Part model, mm, in its own coordinate system. Face numbers are marked on the shaded views. A direction names the side the tool comes from. Give positions to 0.01 mm unless a question says otherwise; leave off trailing zeros. Order: outer loops, then holes, each group sorted by start corner. A loop starts at its lowest first (then second) coordinate and runs counter-clockwise, first axis right, second up.
1. Probe line 1 (Y direction, x = 8, z = 2); line 2 (Y direction, x = 31, z = 9); line 3 (X direction, y = -7.5, z = 8.75). List the from-to ranges inside material, lowest first.
2. Drop flat-ended pins along their axis: pin 1 Ø2.5 at (x, y) = (15, 0) entering from +Z; pin 2 Ø5 at (x, z) = (50, 2.5) entering from -Y; pin 3 Ø1 at (y, z) = (2.5, 7) entering from -X; pin 4 Ø1 at (y, z) = (4.5, 2) entering from -X. Give the stop position or say it passes through.
3. Slice it at B-B on y = 0. List the corners of the cut face in (x, z), and give its area (3 significant figures).
4. Slice it at D-D on y = 7. List the corners of the cut face in (x, z), and give its area (3 significant figures).
5. Slice it at C-C on z = 2. List the corners of the cut face in (x, y).
6. Slice it at A-A on x = 72. List the corners of the cut face in (y, z), and give its area (3 significant figures).
7. Which spindle directions (+Z, -Z, +X, -X, +Y, -Y) get a long thin tool onto all of the face, cutting with end or side? Do the marked faces 1, 2 and 3. Say none if no direction does.
from build123d import *

# Parameters (mm, degrees)
SKETCH1_R           = 1.6
SKETCH1_R_2         = 1.55
BOSS_EXTRUDE1_DEPTH = 10


with BuildPart() as part:
    # Sketch1 → Boss-Extrude1 (new body)
    with BuildSketch(Plane.XY):
        with BuildLine():
            Line((82, 8), (82, -8))
            Line((82, -8), (15.549834435, -8))
            ThreePointArc((15.549834435, -8), (-3, 0), (15.549834435, 8))
            Line((15.549834435, 8), (82, 8))
        make_face()
        with Locations((8, 7)):
            Circle(SKETCH1_R, mode=Mode.SUBTRACT)
        with Locations((1, 0)):
            Circle(SKETCH1_R, mode=Mode.SUBTRACT)
        with Locations((8, -7)):
            Circle(SKETCH1_R, mode=Mode.SUBTRACT)
        with Locations((15, 0)):
            Circle(SKETCH1_R, mode=Mode.SUBTRACT)
        with Locations((8, 0)):
            Circle(SKETCH1_R, mode=Mode.SUBTRACT)
        with Locations((72, 0)):
            Circle(SKETCH1_R_2, mode=Mode.SUBTRACT)
    extrude(amount=BOSS_EXTRUDE1_DEPTH)


solid = part.part
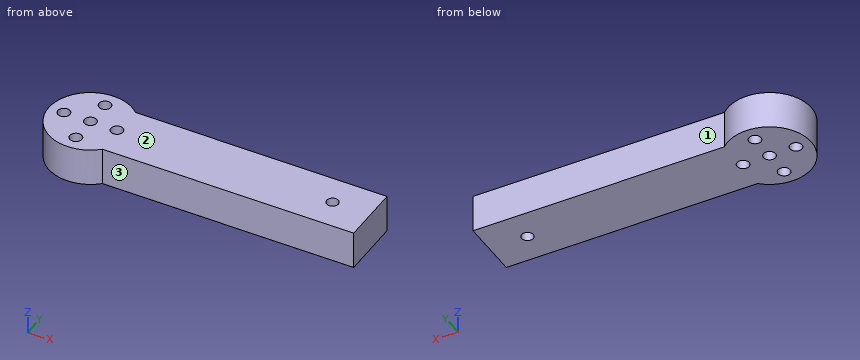
Data:
1. line 1: y = -11 to -8.6, -5.4 to -1.6, 1.6 to 5.4, 8.6 to 11
1. line 2: y = -8 to 8
1. line 3: x = -0.05 to 6.48, 9.52 to 82
2. pin 1: passes through
2. pin 2: stops at y = -8
2. pin 3: stops at x = -2.82
2. pin 4: stops at x = -2.25
3. outline: (-3, 0) - (-0.6, 0) - (-0.6, 10) - (-3, 10) - close; (2.6, 0) - (6.4, 0) - (6.4, 10) - (2.6, 10) - close; (9.6, 0) - (13.4, 0) - (13.4, 10) - (9.6, 10) - close; (16.6, 0) - (70.45, 0) - (70.45, 10) - (16.6, 10) - close; (73.55, 0) - (82, 0) - (82, 10) - (73.55, 10) - close
3. area: 723 mm2
4. outline: (-0.49, 0) - (6.4, 0) - (6.4, 10) - (-0.49, 10) - close; (9.6, 0) - (82, 0) - (82, 10) - (9.6, 10) - close
4. area: 793 mm2
5. outline: (15.55, -8) - (82, -8) - (82, 8) - (15.55, 8) arc R11 ccw (long way) to start; hole circle Ø3.2 at (1, 0); hole circle Ø3.2 at (8, -7); hole circle Ø3.2 at (8, 0); hole circle Ø3.2 at (8, 7); hole circle Ø3.2 at (15, 0); hole circle Ø3.1 at (72, 0)
6. outline: (-8, 0) - (-1.55, 0) - (-1.55, 10) - (-8, 10) - close; (1.55, 0) - (8, 0) - (8, 10) - (1.55, 10) - close
6. area: 129 mm2
7. face 1: +Z, -Z, +X, +Y
7. face 2: +Z, +X, -X, +Y, -Y
7. face 3: +Z, -Z, +X, -Y
